For this review, take the finished solid that the model builds, in its own axes (mm). Face numbers are marked on the shaded views. Coordinates: 2 decimals unless noted, no trailing zeros. Loops run counter-clockwise (first coordinate to the right, second up) from the corner with the lowest first, then second, coordinate; pieces in that order, holes last. Notation, with made-up numbers: M 80,-23 L 100,-23 A25 ccw 100,5 Z; hole C 56,-18.75 d10. An arc over 180 degrees is marked long. Use one line per item in the form item = value.
```python
from build123d import *

# Parameters (mm, degrees)
F0_R     = 49.53
F0_R_2   = 46.99
F1_DEPTH = 63.5
F2_R     = 50.8
F2_R_2   = 49.53
F3_DEPTH = 6.858
F4_SIZE  = 2.54
F5_R     = 1.26999
F6_R     = 50.8
F6_R_2   = 49.53
F7_DEPTH = 6.858
F8_SIZE  = 2.54
F9_R     = 1.26999


# Not quite as in the source:
# - a fillet or chamfer is up to 0.001 mm smaller than in the source, because OpenCascade refuses the exact size


with BuildPart() as f1:
    # F0 (on Top) → F1 (new body)
    with BuildSketch(Plane.XY):
        Circle(F0_R)
        Circle(F0_R_2, mode=Mode.SUBTRACT)
    extrude(amount=F1_DEPTH)

    # F2 (on face) → F3 (join)
    with BuildSketch(Plane.XY.offset(63.5)):
        Circle(F2_R)
        Circle(F2_R_2, mode=Mode.SUBTRACT)
    extrude(amount=-F3_DEPTH)

    # F4
    f4_edges = [f1.edges().sort_by_distance(p)[0] for p in [
        (-50.8, 0, 63.5),
    ]]
    chamfer(f4_edges, length=F4_SIZE)

    # F5 (radius 1.27 in the source; OpenCascade refuses exactly that, so slightly less here)
    f5_edges = [f1.edges().sort_by_distance(p)[0] for p in [
        (-50.8, 0, 56.642),
    ]]
    fillet(f5_edges, radius=F5_R)

    # F6 (on face) → F7 (join)
    with BuildSketch(Plane(origin=(0, 0, 0), x_dir=(1, 0, 0), z_dir=(0, 0, -1))):
        Circle(F6_R)
        Circle(F6_R_2, mode=Mode.SUBTRACT)
    extrude(amount=-F7_DEPTH)

    # F8
    f8_edges = [f1.edges().sort_by_distance(p)[0] for p in [
        (-50.8, 0, 0),
    ]]
    chamfer(f8_edges, length=F8_SIZE)

    # F9 (radius 1.27 in the source; OpenCascade refuses exactly that, so slightly less here)
    f9_edges = [f1.edges().sort_by_distance(p)[0] for p in [
        (-50.8, 0, 6.858),
    ]]
    fillet(f9_edges, radius=F9_R)


solid = f1.part
```
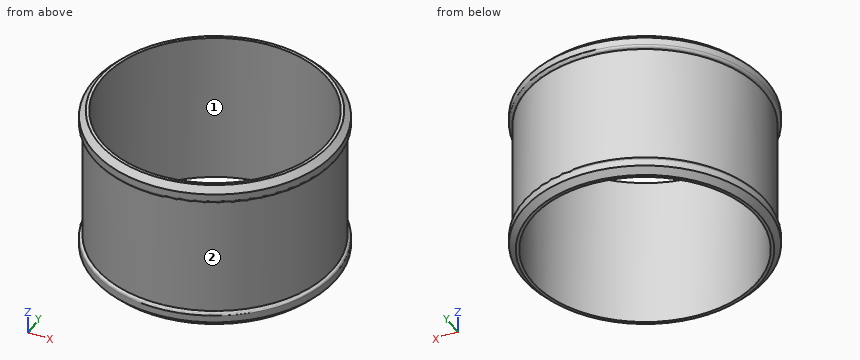
1. For pin 1 Ø12 at (x, z) = (39.5, 49) entering from +Y; pin 2 Ø2 at (y, z) = (-2.5, 6.5) entering from -X; pin 3 Ø12 at (x, y) = (40, 27.5) entering from +Z; pin 4 Ø8 at (x, z) = (-32, 54.5) entering from +Y, all flat-tipped, find the tip position at first contact; note any pin that passes through.
Computed values:
pin_1 = 36.48
pin_2 = -50.76
pin_3 = 63.5
pin_4 = 41.42
2. Draft analysis for pull direction Y (two halves, no side actions). For the marked faces 1 and 2, state which applies: +Y half, -Y half, draft (parallel to the pull), parting line (faces both ways), or undercut.
Computed values:
face_1 = undercut
face_2 = parting line
3. Consider section C-C on z = 25. Write out the cut boundary in (x, y), plus the area to 3 significant figures.
Computed values:
outline = C 0,0 d99.06; hole C 0,0 d93.98
area = 770 mm2
4. Wall thickness on line 1 along Y through (x, z) = (0, 38); line 2 along Y through (x, z) = (-21, 39); line 3 along Z through (x, y) = (-33, -37): over which ranges is each line inside the solid? List them lowest first. Write a range as from..to.
Computed values:
line_1 = -49.53..-46.99, 46.99..49.53
line_2 = -44.86..-42.04, 42.04..44.86
line_3 = 1.32..6.86, 56.64..62.18
